For this review, use the dimensioned drawing (mm, ordinates from the lowest corner) and the shaded views. A direction names the side the tool comes from. Give positions to 0.01 mm unless a question says otherwise; leave off trailing zeros. Order: outer loops, then holes, each group sorted by start corner. A loop starts at its lowest first (then second) coordinate and runs counter-clockwise, first axis right, second up. Notation, with made-up numbers: (74.5, 16.25) -> (121.5, 16.25) arc R23 cw to (121.5, 48.25) -> close; hole circle Ø9 at (42, 21.25). An arc over 180 degrees is marked (long way). One line per item, written item: value. Start each with the question number.
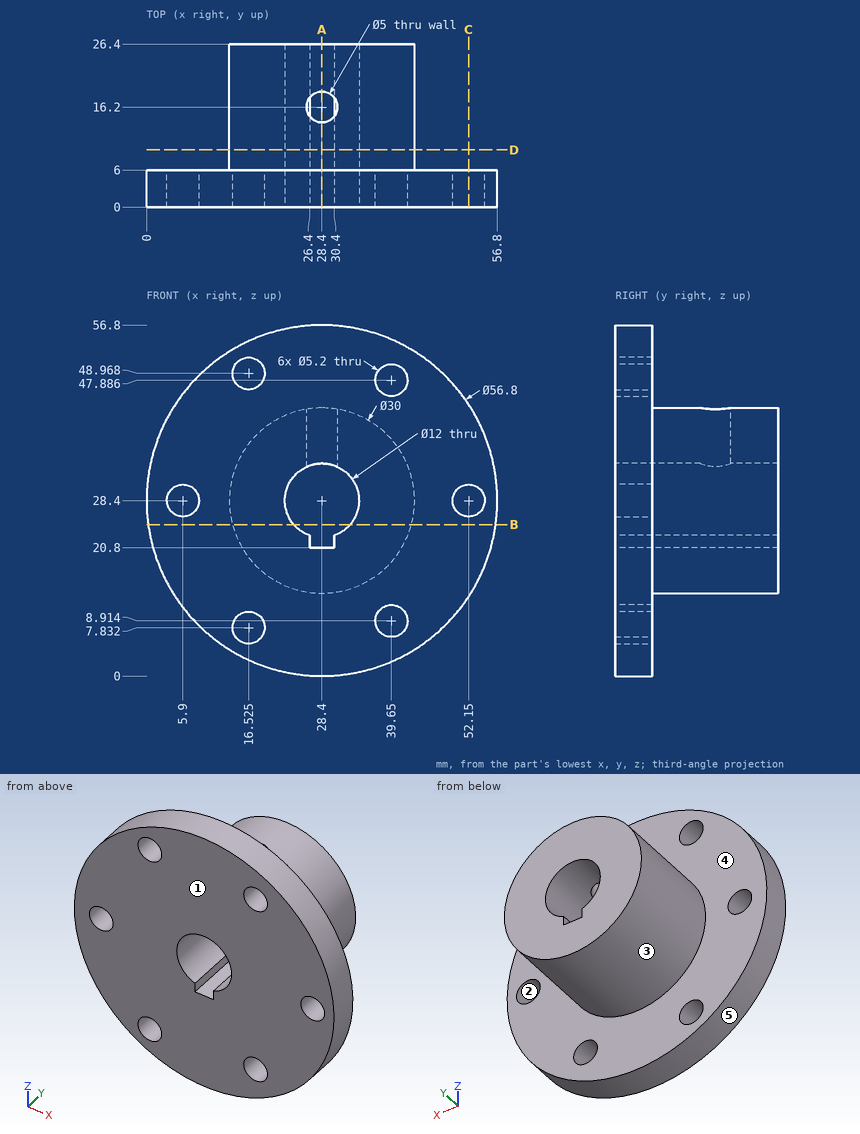
Q1. Take a section at B-B (z = 24.5). State the section outline as (x, y) points.
Q2. For line 1 along X through (y, z) = (22, 28) (1 decimal); line 2 along Y through (x, z) = (15, 20); line 3 along X through (y, z) = (4.75, 21), list the stretches that pass through material, from the lowest coordinate up.
Q3. Mouldability with a two-part tool opening along X and no side actions: class the marked faces 1, 2 and 3 as pulls with the +X half, pulls with the -X half, needs draft (parallel to the pull), parting line crosses it, or undercut.
Q4. Take a section at A-A (x = 28.4). State the section outline as (y, z) points.
Q5. For pin 1 Ø3 at (x, y) = (25, 10) entering from -Z; pin 2 Ø1.5 at (y, z) = (12, 21.5) entering from +X; pin 3 Ø3 at (y, z) = (23.5, 39.5) entering from -X (1 decimal), all flat-tipped, find the tip position at first contact; note any pin that passes through.
Q6. Take a section at C-C (x = 52.15). State the section outline as (y, z) points, and give its area (3 significant figures).
Q7. For the marked faces 4 and 5, list the 3-axis set-ups (+Z, -Z, +X, -X, +Y, -Y) from which the entire face can be reached by the end or side of a thin tool; tool diameter is ignored.
Q8. Take a section at D-D (y = 9.25). State the section outline as (x, z) points.
Answers below:
1. outline: (0.27, 0) -> (23.84, 0) -> (23.84, 26.4) -> (13.92, 26.4) -> (13.92, 6) -> (0.27, 6) -> close; (32.96, 0) -> (56.53, 0) -> (56.53, 6) -> (42.88, 6) -> (42.88, 26.4) -> (32.96, 26.4) -> close
2. line 1: x = 13.4 to 22.4, 34.4 to 43.4
2. line 2: y = 0 to 6
2. line 3: x = 0.98 to 26.4, 30.4 to 55.82
3. face 1: needs draft
3. face 2: undercut
3. face 3: parting line crosses it
4. outline: (0, 0) -> (6, 0) -> (6, 13.4) -> (26.4, 13.4) -> (26.4, 20.8) -> (0, 20.8) -> close; (0, 34.4) -> (13.7, 34.4) -> (13.7, 43.4) -> (6, 43.4) -> (6, 56.8) -> (0, 56.8) -> close; (18.7, 34.4) -> (26.4, 34.4) -> (26.4, 43.4) -> (18.7, 43.4) -> close
5. pin 1: stops at z = 13.52
5. pin 2: stops at x = 42.08
5. pin 3: stops at x = 16.9
6. outline: (0, 12.83) -> (6, 12.83) -> (6, 25.8) -> (0, 25.8) -> close; (0, 31) -> (6, 31) -> (6, 43.97) -> (0, 43.97) -> close
6. area: 156 mm²
7. face 4: +Y
7. face 5: +Y, -Y
8. outline: circle Ø30 at (28.4, 28.4); hole (26.4, 20.8) -> (30.4, 20.8) -> (30.4, 22.74) arc R6 ccw (long way) to (26.4, 22.74) -> close
